```python
from build123d import *

# Parameters (mm, degrees)
PAD_DEPTH    = 10
SKETCH001_W  = 9.110509
SKETCH001_H  = 17.177114
POCKET_DEPTH = 48.001


with BuildPart() as part:
    # Sketch → Pad (new body)
    with BuildSketch(Plane.XY):
        with BuildLine():
            Line((24, 0), (24, -14.5))
            ThreePointArc((22, -16.5), (23.414214, -15.914214), (24, -14.5))
            Line((22, -16.5), (19, -16.5))
            ThreePointArc((18, -15.5), (18.292893, -16.207107), (19, -16.5))
            Line((18, -15.5), (18, -13.5))
            Line((18, -13.5), (21, -13.5))
            Line((21, -13.5), (21, -3))
            Line((21, -3), (-21, -3))
            Line((-21, -3), (-21, -13.5))
            Line((-21, -13.5), (-18, -13.5))
            Line((-18, -13.5), (-18, -15.492764))
            ThreePointArc((-19.00721, -16.492738), (-18.295447, -16.202415), (-18, -15.492764))
            Line((-19.00721, -16.492738), (-22.01442, -16.471056))
            ThreePointArc((-24, -14.471108), (-23.419303, -15.880214), (-22.01442, -16.471056))
            Line((-24, -14.471108), (-24, 0))
            ThreePointArc((-3.646217, 6.4), (-14.188669, 4.362584), (-24, 0))
            ThreePointArc((-3.479417, 4.95934), (-2.869427, 5.759951), (-3.646217, 6.4))
            ThreePointArc((-3.479417, 4.95934), (-12.488364, 3.35813), (-21, 0))
            Line((-21, 0), (21, 0))
            ThreePointArc((21, 0), (12.488364, 3.35813), (3.479417, 4.95934))
            ThreePointArc((3.646217, 6.4), (2.869427, 5.759951), (3.479417, 4.95934))
            ThreePointArc((24, 0), (14.188669, 4.362584), (3.646217, 6.4))
        make_face()
    extrude(amount=PAD_DEPTH)

    # Sketch001 (on Face16 of Pad) → Pocket (cut, through all)
    with BuildSketch(Plane(origin=(-24, 0, 0), x_dir=(0, -1, 0), z_dir=(-1, 0, 0))):
        with Locations((-4.555255, 16.023105)):
            Rectangle(SKETCH001_W, SKETCH001_H)
    extrude(amount=-POCKET_DEPTH, mode=Mode.SUBTRACT)


solid = part.part
```
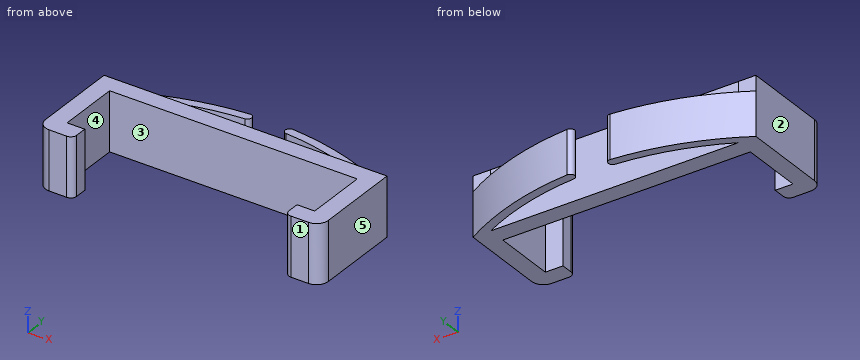
Geometry check sheet. Reference: the model listing, model coordinates, mm. Face numbers are marked on the shaded views. A direction names the side the tool comes from. Coordinates: 2 decimals unless noted, no trailing zeros. Order: outer loops, then holes, each group sorted by start corner. A loop starts at its lowest first (then second) coordinate and runs counter-clockwise, first axis right, second up.
Item 1: Section check C-C (z = 6). Enter the section's corners in (x, y), plus the area to 3 significant figures.
Item 2: Section check A-A (y = -14). Enter the section's corners in (x, z).
Item 3: Depth check by flat-ended pin: pin 1 (2.5 mm diameter, centred on x = 19.5, z = 6.5, fed in from +Y); pin 2 (3 mm diameter, centred on x = 0.5, z = 3.5, fed in from -Y); pin 3 (1.5 mm diameter, centred on x = -20, z = 5, fed in from +Y). Enter the tip coordinate at first touch or a pass-through.
Item 4: Tool access check on the marked faces 4 and 5. Record the directions out of +Z, -Z, +X, -X, +Y, -Y that give a thin tool (end or side, any length) a straight path to the whole face; none if there is none.
Item 5: Section check B-B (x = 16.5). Enter the section's corners in (y, z).
Item 6: Mould release check, pull along X, two halves, no side actions. Record for the marked faces 1, 2 and 3: released by +X, released by -X, zero draft, split by the parting line, or undercut.
Item 7: Scan lines: line 1 along X through (y, z) = (-11, 1.25); line 2 along X through (y, z) = (-14, 3.5); line 3 along Y through (x, z) = (-20.5, 5.5). Record each from-to range of solid material in increasing order.
Check sheet entries:
1. outline: (-24, -14.47) arc R2 ccw to (-22.01, -16.47) - (-19.01, -16.49) arc R1 ccw to (-18, -15.49) - (-18, -13.5) - (-21, -13.5) - (-21, -3) - (21, -3) - (21, -13.5) - (18, -13.5) - (18, -15.5) arc R1 ccw to (19, -16.5) - (22, -16.5) arc R2 ccw to (24, -14.5) - (24, 0) arc R47.3 ccw to (3.65, 6.4) arc R0.73 ccw to (3.48, 4.96) arc R45.85 cw to (21, 0) - (-21, 0) arc R45.85 cw to (-3.48, 4.96) arc R0.73 ccw to (-3.65, 6.4) arc R47.3 ccw to (-24, 0) - close
1. area: 300 mm2
2. outline: (-24, 0) - (-18, 0) - (-18, 10) - (-24, 10) - close; (18, 0) - (24, 0) - (24, 10) - (18, 10) - close
3. pin 1: stops at y = 2.88
3. pin 2: stops at y = -3
3. pin 3: stops at y = 2.45
4. face 4: +Z, -Z
4. face 5: +Z, -Z, +X, +Y, -Y
5. outline: (-3, 0) - (0, 0) - (0, 10) - (-3, 10) - close; (2.02, 0) - (3.57, 0) - (3.57, 7.43) - (2.02, 7.43) - close
6. face 1: zero draft
6. face 2: released by -X
6. face 3: undercut
7. line 1: x = -24 to -21, 21 to 24
7. line 2: x = -24 to -18, 18 to 24
7. line 3: y = -16.48 to -13.5, -3 to 0, 0.25 to 1.87
